```python
from build123d import *

# Parameters (mm, degrees)
SKETCH1_R           = 15
BOSS_EXTRUDE1_DEPTH = 75
SKETCH2_R           = 8.2
CUT_EXTRUDE1_DEPTH  = 5.2
CUT_EXTRUDE2_DEPTH  = 25
SKETCH5_R           = 1.4
CUT_EXTRUDE4_DEPTH  = 14
SKETCH6_R           = 5.5
CUT_EXTRUDE5_DEPTH  = 25
CUT_EXTRUDE6_DEPTH  = 10


with BuildPart() as part:
    # Sketch1 → Boss-Extrude1 (new body)
    with BuildSketch(Plane.XY):
        Circle(SKETCH1_R)
    extrude(amount=BOSS_EXTRUDE1_DEPTH)

    # Sketch2 → Cut-Extrude1 (cut)
    with BuildSketch(Plane.XY.offset(75)):
        Circle(SKETCH2_R)
    extrude(amount=-CUT_EXTRUDE1_DEPTH, mode=Mode.SUBTRACT)

    # Sketch3 → Cut-Extrude2 (cut)
    with BuildSketch(Plane(origin=(0, 0, 0), x_dir=(-1, 0, 0), z_dir=(0, 0, -1))):
        with BuildLine():
            Line((-2.25, 1.089724736), (-2.25, -1.089724736))
            ThreePointArc((-2.25, -1.089724736), (2.5, 0), (-2.25, 1.089724736))
        make_face()
    extrude(amount=-CUT_EXTRUDE2_DEPTH, mode=Mode.SUBTRACT)

    # Sketch5 → Cut-Extrude4 (cut)
    with BuildSketch(Plane(origin=(15, 0, 0), x_dir=(0, 0, -1), z_dir=(1, 0, 0))):
        with Locations((-7, 0)):
            Circle(SKETCH5_R)
    extrude(amount=-CUT_EXTRUDE4_DEPTH, mode=Mode.SUBTRACT)

    # Sketch6 → Cut-Extrude5 (cut)
    with BuildSketch(Plane.XY.offset(69.8)):
        Circle(SKETCH6_R)
    extrude(amount=-CUT_EXTRUDE5_DEPTH, mode=Mode.SUBTRACT)

    # Sketch8 → Cut-Extrude6 (cut)
    with BuildSketch(Plane(origin=(0, 0, 0), x_dir=(-1, 0, 0), z_dir=(0, 0, -1))):
        with BuildLine():
            Line((-2.25, 1.089724736), (-2.25, -1.089724736))
            ThreePointArc((-2.25, -1.089724736), (-2.5, 0), (-2.25, 1.089724736))
        make_face()
    extrude(amount=-CUT_EXTRUDE6_DEPTH, mode=Mode.SUBTRACT)


solid = part.part
```
The listing builds one solid part. Answer for the finished solid, in the listing's coordinates (mm). A direction names the side the tool comes from. Give positions to 0.01 mm unless a question says otherwise; leave off trailing zeros. Write each loop counter-clockwise with the first axis right and the second up, starting at its lowest first coordinate (ties: lowest second). Pieces come first, ordered by that corner, then holes. Notation, with made-up numbers: (66.5, -39.5) - (93.5, -39.5) arc R23 cw to (93.5, -18.5) - close; hole circle Ø8 at (82, 8.25). An arc over 180 degrees is marked (long way). Use one line per item in the form item = value. Start each with the question number.
1) A tool of negligible diameter and unlimited length cuts with its end or side. For faces 5 (the face through (8.63, 0.06, 8.4)), 6 (the face through (2.25, 0, 17)), 7 (the face through (0, 0, 44.8)), from which of +Z, -Z, +X, -X, +Y, -Y can it reach the whole face along a straight path? Write none if from no direction.
2) The mould has two halves that part along Y. Classify faces 1 (the face through (1.7, -5.4, 69.8)), 2 (the face through (6, -6, 75)), 3 (the face through (-14.985, 0.66, 36.975)), 4 (the face through (-1.19, -5.37, 57.47)): pulls with the +Y half, pulls with the -Y half, needs draft (parallel to the pull), parting line crosses it, or undercut.
3) Find section A-A on y = 0. Determine the outline of the cut face in (x, z), plus the area to 3 significant figures.
4) Find section B-B on x = 0. Determine the outline of the cut face in (y, z), plus the area to 3 significant figures.
5) Flat-ended cylindrical pins translate along their axes: pin 1 Ø10 at (y, z) = (-11.5, 11) entering from +X; pin 2 Ø12 at (y, z) = (-9.5, 9.5) entering from -X; pin 3 Ø9 at (x, y) = (-0.5, 0) entering from +Z. Find the tip coordinate at first contact, or state that the pin passes through.
6) Consider line 1 along Z through (x, y) = (6.75, 0); line 2 along Y through (x, z) = (0, 61.25); line 3 along Z through (x, y) = (-8, -1.5). Determine where each line is inside the solid, lowest interval first. Write a range as from..to.
7) Find section C-C on z = 32.5. Determine the outline of the cut face in (x, y).
8) Find section D-D on y = -6.5. Determine the outline of the cut face in (x, z), plus the area to 3 significant figures.
Geometry results:
q1.face_5 = +X
q1.face_6 = -Z
q1.face_7 = +Z
q2.face_1 = undercut
q2.face_2 = needs draft
q2.face_3 = parting line crosses it
q2.face_4 = undercut
q3.outline = (-15, 0) - (-2.5, 0) - (-2.5, 25) - (2.25, 25) - (2.25, 10) - (2.5, 10) - (2.5, 8.4) - (15, 8.4) - (15, 75) - (8.2, 75) - (8.2, 69.8) - (5.5, 69.8) - (5.5, 44.8) - (-5.5, 44.8) - (-5.5, 69.8) - (-8.2, 69.8) - (-8.2, 75) - (-15, 75) - close; (2.5, 0) - (15, 0) - (15, 5.6) - (2.5, 5.6) - close
q3.area = 1,730 mm2
q4.outline = (-15, 0) - (-2.5, 0) - (-2.5, 25) - (2.5, 25) - (2.5, 0) - (15, 0) - (15, 75) - (8.2, 75) - (8.2, 69.8) - (5.5, 69.8) - (5.5, 44.8) - (-5.5, 44.8) - (-5.5, 69.8) - (-8.2, 69.8) - (-8.2, 75) - (-15, 75) - close
q4.area = 1,760 mm2
q5.pin_1 = 13.52
q5.pin_2 = -14.59
q5.pin_3 = 44.8
q6.line_1 = 0..5.6, 8.4..69.8
q6.line_2 = -15..-5.5, 5.5..15
q6.line_3 = 0..69.8
q7.outline = circle Ø30 at (0, 0)
q8.outline = (-13.52, 0) - (13.52, 0) - (13.52, 75) - (5, 75) - (5, 69.8) - (-5, 69.8) - (-5, 75) - (-13.52, 75) - close
q8.area = 1,980 mm2
